Answer from the drawing. Dimensions are ordinates in mm from the lowest x, y and z of the part. Round coordinates to 2 decimals unless told otherwise and drop trailing zeros. Order: outer loops, then holes, each group sorted by start corner. A loop starts at its lowest first (then second) coordinate and runs counter-clockwise, first axis right, second up. Notation, with made-up numbers: (-26, 16.5) -> (-3, 16.5) arc R17 ccw to (-3, 41.5) -> close; hole circle Ø11 at (71, 80.5). An arc over 180 degrees is marked (long way). Use a Markdown table: item, result. Add a question column.
Item 1: A cutting plane is placed at A-A, the plane y = 9.5. Determine the outline of the cut face in (x, z).
Item 2: A cutting plane is placed at B-B, the plane z = 58.5. Determine the outline of the cut face in (x, y).
Item 3: Flat-ended cylindrical pins translate along their axes: P1, Ø2, axis at y = 1.5, z = 117, coming from the -X side; P2, Ø1.2, axis at x = 15, y = 3, coming from the -Z side; P3, Ø3.5, axis at x = 8.5, z = 90, coming from the +Y side; P4, Ø2.5, axis at x = 14.2, y = 3, coming from the +Z side. Find the tip coordinate at first contact, or state that the pin passes through.
Item 4: A cutting plane is placed at C-C, the plane x = 3. Determine the outline of the cut face in (y, z).
Item 5: Find the intervals of material crossed by L1, parallel to Y at x = 3, z = 6.25; L2, parallel to X at y = 10.25, z = 69; L3, parallel to Y at x = 9.25, z = 62, in increasing order. Write a range as [from, to].
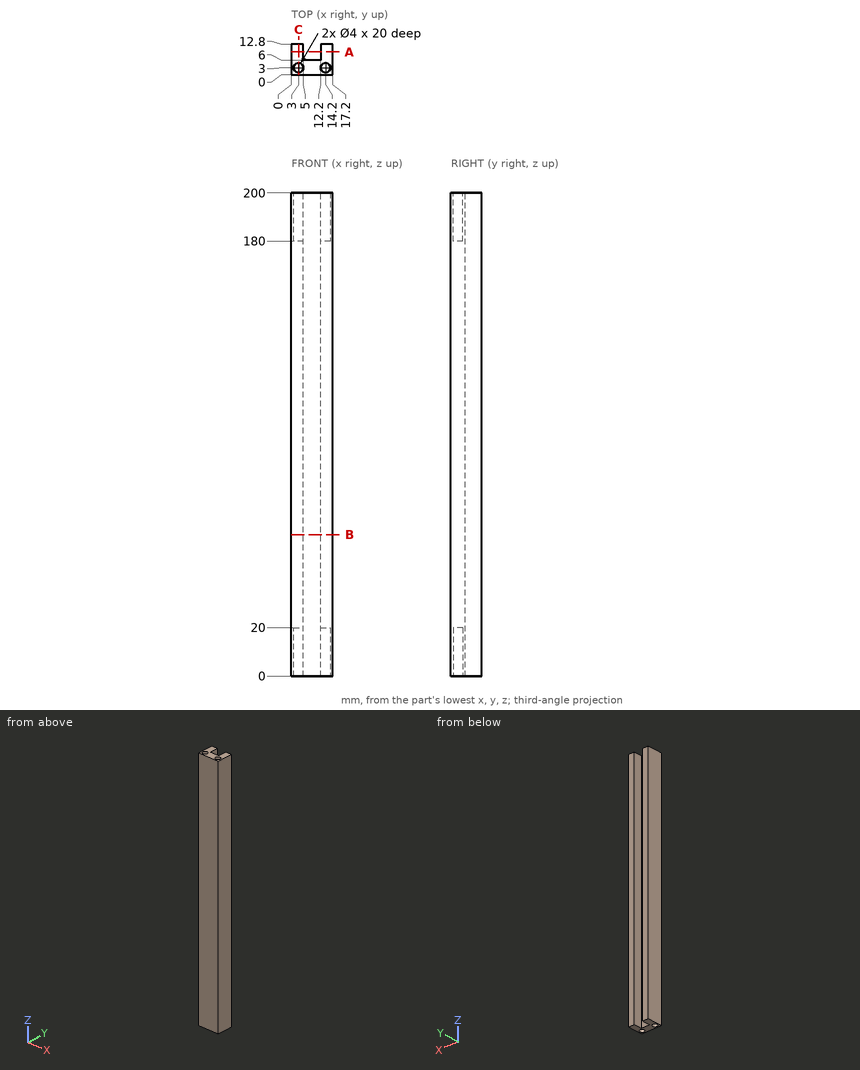
Reported:
| question | item | result |
|---|---|---|
| 1 | outline | (0, 0) -> (5, 0) -> (5, 200) -> (0, 200) -> close; (12.2, 0) -> (17.2, 0) -> (17.2, 200) -> (12.2, 200) -> close |
| 2 | outline | (0, 0) -> (17.2, 0) -> (17.2, 12.8) -> (12.2, 12.8) -> (12.2, 6) -> (5, 6) -> (5, 12.8) -> (0, 12.8) -> close |
| 3 | P1 | x = 0 |
| 3 | P2 | z = 20 |
| 3 | P3 | y = 6 |
| 3 | P4 | z = 180 |
| 4 | outline | (0, 0) -> (1, 0) -> (1, 20) -> (5, 20) -> (5, 0) -> (12.8, 0) -> (12.8, 200) -> (5, 200) -> (5, 180) -> (1, 180) -> (1, 200) -> (0, 200) -> close |
| 5 | L1 | [0, 1], [5, 12.8] |
| 5 | L2 | [0, 5], [12.2, 17.2] |
| 5 | L3 | [0, 6] |
